Here's how the part is built. I have some questions about the finished solid (model axes, mm). Face numbers are marked on the shaded views. A direction names the side the tool comes from. Give positions to 0.01 mm unless a question says otherwise; leave off trailing zeros. Order: outer loops, then holes, each group sorted by start corner. A loop starts at its lowest first (then second) coordinate and runs counter-clockwise, first axis right, second up. Notation, with made-up numbers: (1.5, 74.25) -> (40.5, 74.25) arc R35 ccw to (40.5, 109.25) -> close; hole circle Ø3 at (-5.75, -38.5). An arc over 180 degrees is marked (long way). Write each question's results on one line, items separated by ' | '. Start each with the question number.
Q1. Imagine slicing it at C-C, the plane y = 12. Please give me the cut outline in (x, z), then the cut area to 3 significant figures.
Q2. Imagine slicing it at D-D, the plane y = 6.5. Please give me the cut outline in (x, z).
Q3. Imagine slicing it at B-B, the plane z = 0.3. Please give me the cut outline in (x, y).
Q4. For the marked faces 1 and 2, which set-ups out of +Z, -Z, +X, -X, +Y, -Y let a thin tool reach every point of the face, with its end or its side?
Q5. I need wall thicknesses on line 1 along Z through (x, y) = (0, 2.95); line 2 along Y through (x, z) = (-1.15, -1.2); line 3 along Z through (x, y) = (1.65, 9.25). Which ranges of each line are inside material? Lowest first, please. Write a range as [from, to].
Q6. I'm going to push flat-ended pins straight in: pin 1 (2 mm diameter, centred on x = 0.5, z = 0.5, fed in from -Y); pin 2 (1.5 mm diameter, centred on y = 9, z = -1.5, fed in from -X); pin 3 (1.5 mm diameter, centred on y = 11, z = -0.5, fed in from -X); pin 4 (2 mm diameter, centred on x = 1.5, y = 11.5, fed in from -Z). Where does each tip first touch, or does it pass through?
Q7. Thinking about a two-plate mould opening in X: for the marked faces 3, 4 and 5, which applies, pulls with the +X half, pulls with the -X half, needs draft (parallel to the pull), parting line crosses it, or undercut?
Q8. Imagine slicing it at A-A, the plane x = 0. Please give me the cut outline in (y, z), then the cut area to 3 significant figures.
Autodesk Inventor part; units mm, degrees
ref_plane "YZ Plane" through (0, 0, 0) normal (1, 0, 0) x (0, 1, 0)
ref_plane "XZ Plane" through (0, 0, 0) normal (0, 1, 0) x (-1, 0, 0)
ref_plane "XY Plane" through (0, 0, 0) normal (0, 0, 1) x (1, 0, 0)
sketch "Sketch1" plane through (0, 0, 0) normal (0, 1, 0) x (-1, 0, 0)
  line L0 (2.3094, 0) -> (1.1547, -2)
  line L1 (1.1547, -2) -> (-1.1547, -2)
  line L2 (-1.1547, -2) -> (-2.3094, 0)
  line L3 (-2.3094, 0) -> (-1.1547, 2)
  line L4 (-1.1547, 2) -> (1.1547, 2)
  line L5 (1.1547, 2) -> (2.3094, 0)
  point P0 (0, 0)
  point P1 (0, 0)
  dimension "d0" = 4
extrude "Extrusion1" add sketch "Sketch1" along normal blind 10
sketch "Sketch2" plane through (0, 10, 0) normal (0, 1, 0) x (1, 0, 0)
  circle A0 centre (0, 0) radius 1
  dimension "d3" = 2
extrude "Extrusion2" add sketch "Sketch2" along normal blind 5
sketch "Sketch3" plane through (0, 0, 0) normal (0, -1, 0) x (1, 0, 0)
  circle A0 centre (0, 0) radius 1
  dimension "d6" = 2
extrude "Extrusion3" cut sketch "Sketch3" against normal blind 6
properties part number "M2x12 HEX SPACER"
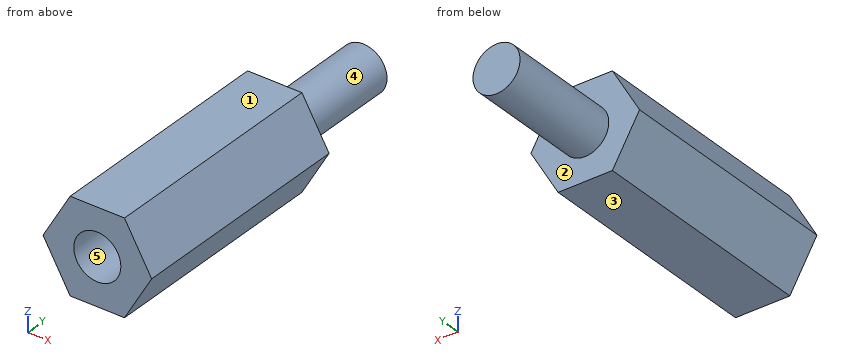
Geometry check:
1) outline: circle Ø2 at (0, 0) | area: 3.14 mm²
2) outline: (-2.31, 0) -> (-1.15, -2) -> (1.15, -2) -> (2.31, 0) -> (1.15, 2) -> (-1.15, 2) -> close
3) outline: (-2.14, 0) -> (-0.95, 0) -> (-0.95, 6) -> (0.95, 6) -> (0.95, 0) -> (2.14, 0) -> (2.14, 10) -> (0.95, 10) -> (0.95, 15) -> (-0.95, 15) -> (-0.95, 10) -> (-2.14, 10) -> close
4) face 1: +Z, +X, -X, +Y, -Y | face 2: +Y
5) line 1: [-2, -1], [1, 2] | line 2: [0, 10] | line 3: [-1.14, 1.14]
6) pin 1: y = 0 | pin 2: x = -1.88 | pin 3: x = -1 | pin 4: z = -0.87
7) face 3: needs draft | face 4: parting line crosses it | face 5: undercut
8) outline: (0, -2) -> (10, -2) -> (10, -1) -> (15, -1) -> (15, 1) -> (10, 1) -> (10, 2) -> (0, 2) -> (0, 1) -> (6, 1) -> (6, -1) -> (0, -1) -> close | area: 38.0 mm²
